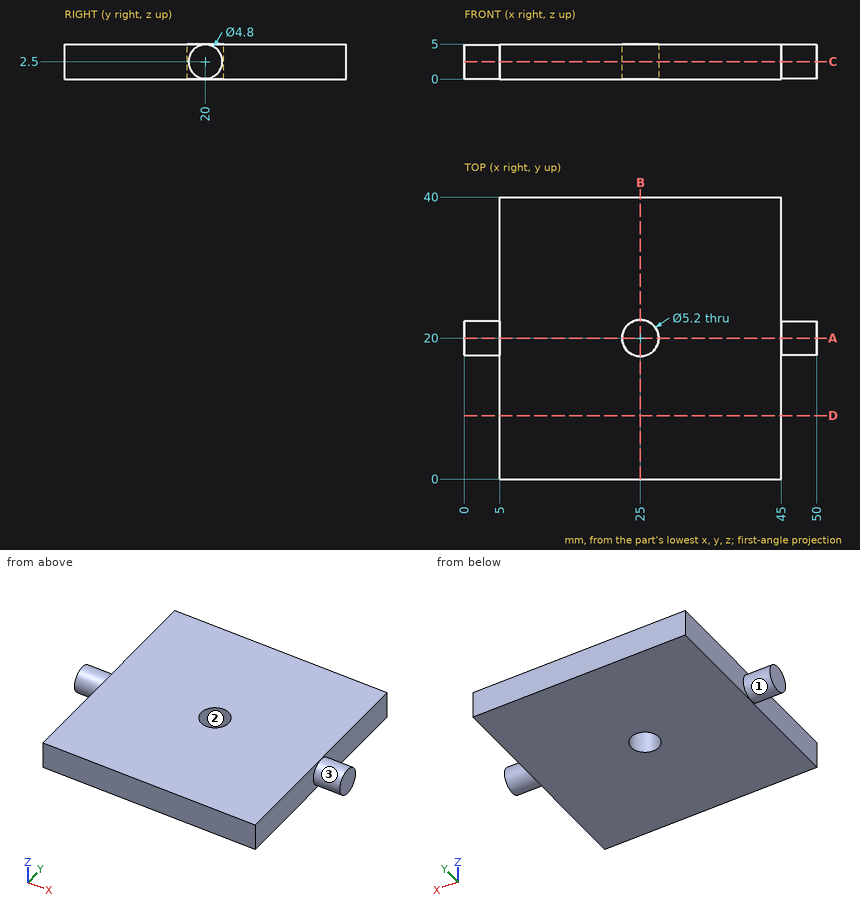
Input: dimensioned drawing with shaded views. Units: mm. Origin: part minimum x, y, z. A direction names the side the tool comes from. Coordinates: 2 decimals unless noted, no trailing zeros. Write each loop counter-clockwise with the first axis right and the second up, starting at its lowest first coordinate (ties: lowest second). Pieces come first, ordered by that corner, then holes. Notation, with made-up numbers: M 89.5,56 L 130.5,56 A25 cw 130.5,94 Z; hole C 44.25,11 d1. An arc over 180 degrees is marked long. Answer as a JSON object with one key per item and string values. Group by question number.
(1) Section A-A on y = 20. Output: boundary loops of the cut face in (x, z), plus the area to 3 significant figures.
(2) Section D-D on y = 9. Output: boundary loops of the cut face in (x, z), plus the area to 3 significant figures.
(3) Section C-C on z = 2.5. Output: boundary loops of the cut face in (x, y).
(4) Section B-B on x = 25. Output: boundary loops of the cut face in (y, z).
(5) Ray query, line 1 along Y through (x, z) = (25, 3.55); line 2 along X through (y, z) = (20, 3); line 3 along X through (y, z) = (16, 1.5). Return the intervals inside material, ascending. Write a range as [from, to].
(6) Set-up query: the marked faces 1, 2 and 3. Return all of +Z, -Z, +X, -X, +Y, -Y with unobstructed straight access to the full face (end or side cutting, diameter ignored); none if empty.
Result set:
{
 "1": {"outline": "M 0,0.1 L 5,0.1 L 5,0 L 22.4,0 L 22.4,5 L 5,5 L 5,4.9 L 0,4.9 Z; M 27.6,0 L 45,0 L 45,0.1 L 50,0.1 L 50,4.9 L 45,4.9 L 45,5 L 27.6,5 Z", "area": "222 mm2"},
 "2": {"outline": "M 5,0 L 45,0 L 45,5 L 5,5 Z", "area": "200 mm2"},
 "3": {"outline": "M 0,17.6 L 5,17.6 L 5,0 L 45,0 L 45,17.6 L 50,17.6 L 50,22.4 L 45,22.4 L 45,40 L 5,40 L 5,22.4 L 0,22.4 Z; hole C 25,20 d5.2"},
 "4": {"outline": "M 0,0 L 17.4,0 L 17.4,5 L 0,5 Z; M 22.6,0 L 40,0 L 40,5 L 22.6,5 Z"},
 "5": {"line 1": "y = [0, 17.4], [22.6, 40]", "line 2": "x = [0, 22.4], [27.6, 50]", "line 3": "x = [5, 45]"},
 "6": {"face 1": "-X", "face 2": "+Z, -Z", "face 3": "+X"}
}
